Design review of the part built by this model. Coordinates are the model's own, in mm. Give positions to 0.01 mm unless a question says otherwise; leave off trailing zeros. Loops run counter-clockwise (first coordinate to the right, second up) from the corner with the lowest first, then second, coordinate; pieces in that order, holes last. Notation, with made-up numbers: (74.25, 69.5) -> (131.25, 69.5) arc R18 ccw to (131.25, 79.5) -> close; hole circle Ø10 at (61.25, 27). An arc over 180 degrees is marked (long way). Use a Markdown table: item, result. Add a question column.
1. To check wall thickness, follow line 1 (X direction, y = -13.97, z = 0.95); line 2 (X direction, y = 2.5, z = 0.2). State the ranges of each line that lie inside material, in increasing order.
2. Add section A-A (y = -1). State the section outline as (x, z) points, and give its area (3 significant figures).
3. Add section B-B (x = 13.97). State the section outline as (y, z) points, and give its area (3 significant figures).
4. Add section D-D (z = 0.2). Count the separate pieces of the cut face and the enclosed holes in it, and give its area (3 significant figures).
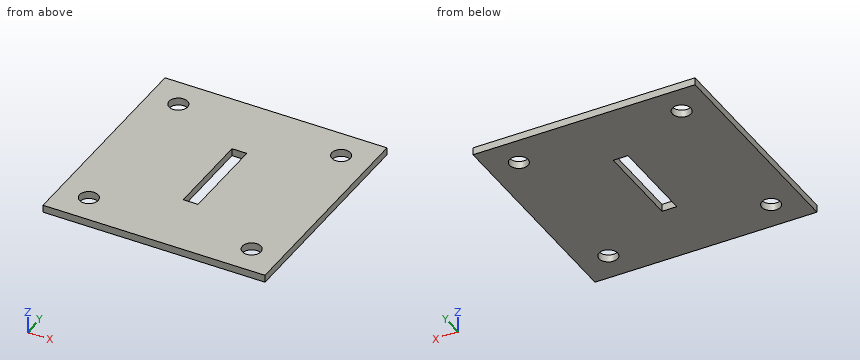
```python
from build123d import *

# Parameters (mm, degrees)
F0_W     = 38.1
F0_H     = 38.1
F1_DEPTH = 1.27
F3_R     = 1.5875
F4_DEPTH = 25.4
F7_W     = 2.54
F7_H     = 15.24
F8_DEPTH = 25.4


with BuildPart() as f1:
    # F0 (on Top) → F1 (new body)
    with BuildSketch(Plane.XY):
        Rectangle(F0_W, F0_H)
    extrude(amount=F1_DEPTH)

    # F3 (on Top) → F4 (cut)
    with BuildSketch(Plane.XY):
        with Locations((13.97, 13.97)):
            Circle(F3_R)
    extrude(amount=F4_DEPTH, mode=Mode.SUBTRACT)

    # F5: F1 across plane


with BuildPart() as f1_1:
    add(f1.part)
    add(f1.part.mirror(Plane.YZ), mode=Mode.INTERSECT)

    # F6: F1 across plane


with BuildPart() as f1_2:
    add(f1_1.part)
    add(f1_1.part.mirror(Plane.XZ), mode=Mode.INTERSECT)

    # F7 (on Top) → F8 (cut)
    with BuildSketch(Plane.XY):
        Rectangle(F7_W, F7_H)
    extrude(amount=F8_DEPTH, mode=Mode.SUBTRACT)


solid = f1_2.part
```
Taken from the geometry:
| question | item | result |
|---|---|---|
| 1 | line 1 | x = -19.05 to -15.56, -12.38 to 12.38, 15.56 to 19.05 |
| 1 | line 2 | x = -19.05 to -1.27, 1.27 to 19.05 |
| 2 | outline | (-19.05, 0) -> (-1.27, 0) -> (-1.27, 1.27) -> (-19.05, 1.27) -> close; (1.27, 0) -> (19.05, 0) -> (19.05, 1.27) -> (1.27, 1.27) -> close |
| 2 | area | 45.2 mm^2 |
| 3 | outline | (-19.05, 0) -> (-15.56, 0) -> (-15.56, 1.27) -> (-19.05, 1.27) -> close; (-12.38, 0) -> (12.38, 0) -> (12.38, 1.27) -> (-12.38, 1.27) -> close; (15.56, 0) -> (19.05, 0) -> (19.05, 1.27) -> (15.56, 1.27) -> close |
| 3 | area | 40.3 mm^2 |
| 4 | separate pieces | 1 |
| 4 | enclosed holes | 5 |
| 4 | area | 1,380 mm^2 |
